from build123d import *

# Parameters (mm, degrees)
F0_R     = 13
F2_R     = 11
F4_R     = 3
F5_R     = 2
F6_DEPTH = 22.001


with BuildPart() as f3:
    # F0 (on Front) → F3 section 0
    with BuildSketch(Plane.XZ):
        Circle(F0_R)
    # F2 (on offset) → F3 section 1
    with BuildSketch(Plane.XZ.offset(22)):
        Circle(F2_R)
    loft()

    # F4
    f4_edges = [f3.edges().sort_by_distance(p)[0] for p in [
        (-11, -22, 0),
    ]]
    fillet(f4_edges, radius=F4_R)

    # F5 (on Front) → F6 (cut, through all)
    with BuildSketch(Plane.XZ):
        Circle(F5_R)
    extrude(amount=F6_DEPTH, mode=Mode.SUBTRACT)


solid = f3.part
Check sheet for the modelled part. Datum: model origin and axes. Units: mm. Round coordinates to 2 decimals unless told otherwise and drop trailing zeros. Write each loop counter-clockwise with the first axis right and the second up, starting at its lowest first coordinate (ties: lowest second). Pieces come first, ordered by that corner, then holes. Notation, with made-up numbers: (-18, 17.5) -> (16, 17.5) arc R21 cw to (16, 51.5) -> close; hole circle Ø6 at (-15.75, -2). An arc over 180 degrees is marked (long way). Answer as CSV lines item,"result". Start each with the question number.
1) Section check B-B on y = -13.5. Enter the section's corners in (x, z), and give its area (3 significant figures).
2) Section check A-A on x = 0. Enter the section's corners in (y, z), and give its area (3 significant figures).
3) Release check for a two-part mould opening along X. For faces 1 (the conical face through (-2.583, -11.912, -11.634)), 2 (the flat face through (3, 0, 0)), 3 (the cylindrical face through (0, -11, -2)) record: pulls with the +X half, pulls with the -X half, needs draft (parallel to the pull), parting line crosses it, or undercut.
4) Go/stop test with flat-tipped pins: P1, Ø8, axis at y = -4, z = 2.5, coming from the -X side; P2, Ø3, axis at y = -16, z = -9.5, coming from the -X side; P3, Ø2, axis at x = 1.5, y = -19.5, coming from the +Z side; P4, Ø1.5, axis at x = 0.5, z = 2, coming from the +Y side. Record where each tip stops, or that it passes through.
5) Material ranges on line 1 (Z direction, x = 1.5, y = -11); line 2 (Z direction, x = 0, y = -10.5); line 3 (X direction, y = -8, z = 0), recorded low to high. Write a range as from..to.
Found:
1,outline,"circle Ø23.55 at (0, 0); hole circle Ø4 at (0, 0)"
1,area,"423 mm^2"
2,outline,"(-22, -8.26) arc R3 ccw to (-19.27, -11.25) -> (0, -13) -> (0, -2) -> (-22, -2) -> close; (-22, 2) -> (0, 2) -> (0, 13) -> (-19.27, 11.25) arc R3 ccw to (-22, 8.26) -> close"
2,area,"437 mm^2"
3,face 1,"parting line crosses it"
3,face 2,"needs draft"
3,face 3,"undercut"
4,P1,"stops at x = -12.94"
4,P2,"stops at x = -8.34"
4,P3,"stops at z = 11.26"
4,P4,"stops at y = 0"
5,line 1,"z = -11.91..-1.32, 1.32..11.91"
5,line 2,"z = -12.05..-2, 2..12.05"
5,line 3,"x = -12.27..-2, 2..12.27"
